The listing builds one solid part. Answer for the finished solid, in the listing's coordinates (mm). Coordinates: 2 decimals unless noted, no trailing zeros. Order: outer loops, then holes, each group sorted by start corner. A loop starts at its lowest first (then second) coordinate and runs counter-clockwise, first axis right, second up. Notation, with made-up numbers: (-20, 71) -> (10, 71) arc R28 cw to (10, 94) -> close; hole circle Ø8 at (56.5, 86.5). An arc over 180 degrees is marked (long way). Return JSON: item names as keys, results as strings.
```python
from build123d import *

# Parameters (mm, degrees)
CHAMFER_1_SIZE           = 1
SKETCH_4_W               = 2
SKETCH_4_H               = 1
CUT_EXTRUDE_1_DEPTH      = 24.334523779
CUT_EXTRUDE_2_REACH      = 25.335
PATTERN_CIRCULAR_3_COUNT = 20
SKETCH_7_R               = 2.8338
CUT_EXTRUDE_3_DEPTH      = 24.27268664
SKETCH_8_R               = 3.6676
CUT_EXTRUDE_4_DEPTH      = 15
SKETCH_9_R               = 2.8338
SKETCH_9_R_2             = 2.5
EXTRUDE_1_DEPTH          = 5


with BuildPart() as part:
    # 草图1 → 旋转1 (revolve)
    with BuildSketch(Plane.XY, mode=Mode.PRIVATE) as revolve_1_sk:
        Polygon((0, 1.8338), (0, 8.5), (5, 8.5), (5, 3.6676), (20, 3.6676), (20, 1.8338), align=None)
    revolve(revolve_1_sk.sketch.rotate(Axis((0, 0, 0), (1, 0, 0)), 90), axis=Axis((0, 0, 0), (1, 0, 0)))

    # 倒角1
    chamfer_1_edges = [part.edges().sort_by_distance(p)[0] for p in [
        (20, 0, -1.8338),
        (0, 0, -1.8338),
    ]]
    chamfer(chamfer_1_edges, length=CHAMFER_1_SIZE)

    # 草图4 → 切除-拉伸1 (cut, through all)
    with BuildSketch(Plane.ZY):
        with Locations((0, 2.037147501)):
            Rectangle(SKETCH_4_W, SKETCH_4_H)
    extrude(amount=-CUT_EXTRUDE_1_DEPTH, mode=Mode.SUBTRACT)

    # 草图6 → 切除-拉伸2 (cut, up to next)
    with BuildSketch(Plane(origin=(0, 0, 0), x_dir=(0, 0, -1), z_dir=(1, 0, 0)), mode=Mode.PRIVATE) as cut_extrude_2_sk1:
        with BuildLine():
            Line((0.923770376, 8.186492725), (0.903216998, 8.019098898))
            ThreePointArc((0.903216998, 8.019098898), (0, 7.22), (-0.903216998, 8.019098898))
            Line((-0.903216998, 8.019098898), (-0.923770376, 8.186492725))
            ThreePointArc((-0.923770376, 8.186492725), (-1.023997868, 8.36141809), (-1.219123202, 8.412118557))
            ThreePointArc((-1.219123202, 8.412118557), (-1.347636542, 8.392489246), (-1.475834638, 8.370896733))
            Line((-1.475834638, 8.370896733), (-1.672482627, 9.972466076))
            ThreePointArc((-1.672482627, 9.972466076), (0, 10.111739601), (1.672482627, 9.972466076))
            Line((1.672482627, 9.972466076), (1.475834638, 8.370896733))
            ThreePointArc((1.475834638, 8.370896733), (1.347636542, 8.392489246), (1.219123202, 8.412118557))
            ThreePointArc((1.219123202, 8.412118557), (1.023997868, 8.36141809), (0.923770376, 8.186492725))
        make_face()
    cut_extrude_2_tool1 = extrude(cut_extrude_2_sk1.sketch, amount=CUT_EXTRUDE_2_REACH, mode=Mode.PRIVATE) & part.part
    cut_extrude_2 = cut_extrude_2_tool1.solids().sort_by_distance((0, 8.902144, 0))[0]
    add(cut_extrude_2, mode=Mode.SUBTRACT)

    # 阵列(圆周)3: 切除-拉伸2 ×20 about axis
    pattern_circular_3_axis = Axis((0, 0, 0), (1, 0, 0))
    for i in range(1, PATTERN_CIRCULAR_3_COUNT):
        add(cut_extrude_2.rotate(pattern_circular_3_axis, i * 360 / PATTERN_CIRCULAR_3_COUNT), mode=Mode.SUBTRACT)

    # 草图7 → 切除-拉伸3 (cut, through all)
    with BuildSketch(Plane.ZY):
        Circle(SKETCH_7_R)
    extrude(amount=-CUT_EXTRUDE_3_DEPTH, mode=Mode.SUBTRACT)

    # 草图8 → 切除-拉伸4 (cut)
    with BuildSketch(Plane(origin=(20, 0, 0), x_dir=(0, 0, -1), z_dir=(1, 0, 0))):
        Circle(SKETCH_8_R)
    extrude(amount=-CUT_EXTRUDE_4_DEPTH, mode=Mode.SUBTRACT)

    # 草图9 → 凸台-拉伸1 (add)
    with BuildSketch(Plane.ZY):
        Circle(SKETCH_9_R)
        Circle(SKETCH_9_R_2, mode=Mode.SUBTRACT)
    extrude(amount=-EXTRUDE_1_DEPTH)


solid = part.part
```
Item 1: Flat-ended cylindrical pins translate along their axes: pin 1 (1.5 mm diameter, centred on x = 2, y = 5.5, fed in from -Z); pin 2 (1 mm diameter, centred on x = 4, z = -6.5, fed in from -Y); pin 3 (3 mm diameter, centred on x = 4, y = 4.5, fed in from +Z). Find the tip coordinate at first contact, or state that the pin passes through.
Answer list:
{"pin 1": "z = -6.16", "pin 2": "y = -6.02", "pin 3": "z = 7.65"}
Item 2: Determine the mould class of faces 1 (the cylindrical face through (2.46, 0.02, 7.22)), 2 (the cylindrical face through (2.46, -0.02, -7.22)), 3 (the cylindrical face through (2.46, -5.83, 4.26)), 4 (the cylindrical face through (2.46, -4.23, 5.85)) for opening direction Z: pulls with the +Z half, pulls with the -Z half, needs draft (parallel to the pull), parting line crosses it, or undercut.
Answer list:
{"face 1": "pulls with the +Z half", "face 2": "pulls with the -Z half", "face 3": "undercut", "face 4": "undercut"}
Item 3: The part is cut by section A-A on y = 0. Determine the outline of the cut face in (x, z).
Answer list:
{"outline": "(0, -7.22) -> (5, -7.22) -> (5, -2.5) -> (0, -2.5) -> close; (0, 2.5) -> (5, 2.5) -> (5, 7.22) -> (0, 7.22) -> close"}
Item 4: Find the intervals of material crossed by probe 1 along Z at (x, y) = (2.25, -5.75); probe 2 along Y at (x, z) = (4.2, 7); probe 3 along Y at (x, z) = (3.85, 6), in increasing order.
Answer list:
{"probe 1": "-6.16 to -5.16, -4.4 to 4.4, 5.16 to 6.16", "probe 2": "-3.97 to -3.05, -1.97 to 1.97, 3.05 to 3.97", "probe 3": "-6.02 to -5.48, -4.08 to 4.08, 5.48 to 6.02"}
Item 5: The part is cut by section C-C on z = -4.5. Determine the outline of the cut face in (x, y).
Answer list:
{"outline": "(0, -5.71) -> (5, -5.71) -> (5, 5.71) -> (0, 5.71) -> close"}
